Verification items for the finished model (mm, model axes). Face numbers are marked on the shaded views. A direction names the side the tool comes from. Coordinates: 2 decimals unless noted, no trailing zeros. Order: outer loops, then holes, each group sorted by start corner. A loop starts at its lowest first (then second) coordinate and runs counter-clockwise, first axis right, second up. Notation, with made-up numbers: M -29,-13 L 23,-13 A25 cw 23,0 Z; hole C 73.25,-31 d7. An arc over 180 degrees is marked long. Return JSON: item names as keys, results as strings. Group by question number.
Q1. Section check C-C, the plane y = 9. Enter the section's corners in (x, z), then the cut area to 3 significant figures.
Q2. Section check D-D, the plane z = -2.5. Enter the section's corners in (x, y).
Q3. Go/stop test with a flat-tipped pin: pin 1 Ø3 at (x, y) = (2, 5) entering from -Z. Record where the tip stops, or that it passes through.
Q4. Mould release check, pull along X, two halves, no side actions. Record for the marked faces 3, 4 and 5: pulls with the +X half, pulls with the -X half, needs draft (parallel to the pull), parting line crosses it, or undercut.
Q5. Thickness scan on probe 1 along Y at (x, z) = (-3.75, -1.5); probe 2 along Y at (x, z) = (0, 4.4); probe 3 along Z at (x, y) = (2.25, 7). Record the ranges inside material, lowest first.
Q6. Section check B-B, the plane x = 0. Enter the section's corners in (y, z), then the cut area to 3 significant figures.
Q7. Access from +Z, -Z, +X, -X, +Y, -Y to the whole of each face (thin tool, end or side, straight path). Record for the marked faces 1 and 2.
Q8. Section check A-A, the plane z = 2.5. Enter the section's corners in (x, y).
from build123d import *

# Parameters (mm, degrees)
EXTRUDE_1_DEPTH     = 10
SKETCH_2_W          = 8
SKETCH_2_H          = 6
CUT_EXTRUDE_1_DEPTH = 10
SKETCH_3_R          = 1.75
CUT_EXTRUDE_2_DEPTH = 10
FILLET_1_R          = 1
SKETCH_4_R          = 1.6
CUT_EXTRUDE_3_DEPTH = 10
CHAMFER_1_SIZE      = 1


with BuildPart() as part:
    # 草图1 → 凸台-拉伸1 (new body)
    with BuildSketch(Plane(origin=(0, 0, 0), x_dir=(1, 0, 0), z_dir=(0, 1, 0))):
        Polygon((-2.5, 5), (-5, -1.550851348), (-5, -5), (5, -5), (5, -1.550851348), (2.5, 5), align=None)
    extrude(amount=EXTRUDE_1_DEPTH)

    # 草图2 → 切除-拉伸1 (cut)
    with BuildSketch(Plane(origin=(5, 0, 0), x_dir=(0, 0, -1), z_dir=(1, 0, 0))):
        with Locations((1, 5)):
            Rectangle(SKETCH_2_W, SKETCH_2_H)
    extrude(amount=-CUT_EXTRUDE_1_DEPTH, mode=Mode.SUBTRACT)

    # 草图3 → 切除-拉伸2 (cut)
    with BuildSketch(Plane.XZ):
        with Locations(Location((0, -1, 0), (0, 0, 270))):
            Circle(SKETCH_3_R)
    extrude(amount=-CUT_EXTRUDE_2_DEPTH, mode=Mode.SUBTRACT)

    # 圆角1
    fillet_1_edges = [part.edges().sort_by_distance(p)[0] for p in [
        (-2.5, 9, -5),
        (2.5, 9, -5),
        (-2.5, 1, -5),
        (2.5, 1, -5),
    ]]
    fillet(fillet_1_edges, radius=FILLET_1_R)

    # 草图4 → 切除-拉伸3 (cut)
    with BuildSketch(Plane(origin=(0, 0, 3), x_dir=(-1, 0, 0), z_dir=(0, 0, -1))):
        with Locations((0, 4.900814168)):
            Circle(SKETCH_4_R)
    extrude(amount=-CUT_EXTRUDE_3_DEPTH, mode=Mode.SUBTRACT)

    # 倒角1
    chamfer_1_edges = [part.edges().sort_by_distance(p)[0] for p in [
        (1.6, 4.900814168, 3),
    ]]
    chamfer(chamfer_1_edges, length=CHAMFER_1_SIZE)


solid = part.part
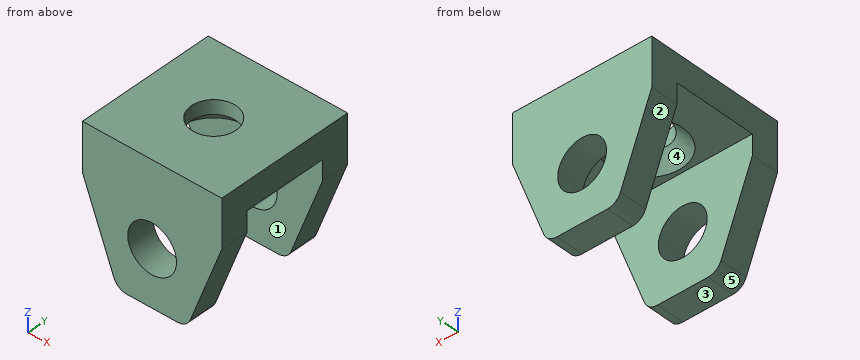
Numbers:
{
 "1": {"outline": "M -5,1.55 L -2.75,-4.36 A1 ccw -1.81,-5 L 1.81,-5 A1 ccw 2.75,-4.36 L 5,1.55 L 5,5 L -5,5 Z; hole C 0,-1 d3.5", "area": "73.8 mm2"},
 "2": {"outline": "M -3.45,0 L -0.9,0 L -0.9,2 L -3.45,2 Z; M -3.45,8 L -0.9,8 L -0.9,10 L -3.45,10 Z; M 0.9,0 L 3.45,0 L 3.45,2 L 0.9,2 Z; M 0.9,8 L 3.45,8 L 3.45,10 L 0.9,10 Z"},
 "3": {"pin 1": "stops at z = 3"},
 "4": {"face 3": "needs draft", "face 4": "undercut", "face 5": "pulls with the -X half"},
 "5": {"probe 1": "y = 0 to 2, 8 to 10", "probe 2": "y = 0 to 3.3, 6.5 to 10", "probe 3": "z = 3 to 5"},
 "6": {"outline": "M 0,-5 L 2,-5 L 2,-2.75 L 0,-2.75 Z; M 0,0.75 L 2,0.75 L 2,3 L 2.3,3 L 3.3,4 L 3.3,5 L 0,5 Z; M 6.5,4 L 7.5,3 L 8,3 L 8,0.75 L 10,0.75 L 10,5 L 6.5,5 Z; M 8,-5 L 10,-5 L 10,-2.75 L 8,-2.75 Z", "area": "30.6 mm2"},
 "7": {"face 1": "-Z, +X, -X", "face 2": "-Z, -X, +Y, -Y"},
 "8": {"outline": "M -5,0 L 5,0 L 5,2 L -5,2 Z; M -5,8 L 5,8 L 5,10 L -5,10 Z"}
}
